Part print with two shaded views. Sizes in mm from the minimum x, y, z corner. A direction names the side the tool comes from. Give positions to 0.01 mm unless a question says otherwise; leave off trailing zeros. Write each loop counter-clockwise with the first axis right and the second up, starting at its lowest first coordinate (ties: lowest second). Pieces come first, ordered by that corner, then holes. Notation, with made-up numbers: (80, -26.75) - (119, -26.75) arc R19 ccw to (119, -4.75) - close; hole circle Ø6 at (26.25, 41.25). An arc over 180 degrees is marked (long way). Answer as a JSON object with one key per item and string values. Group by question number.
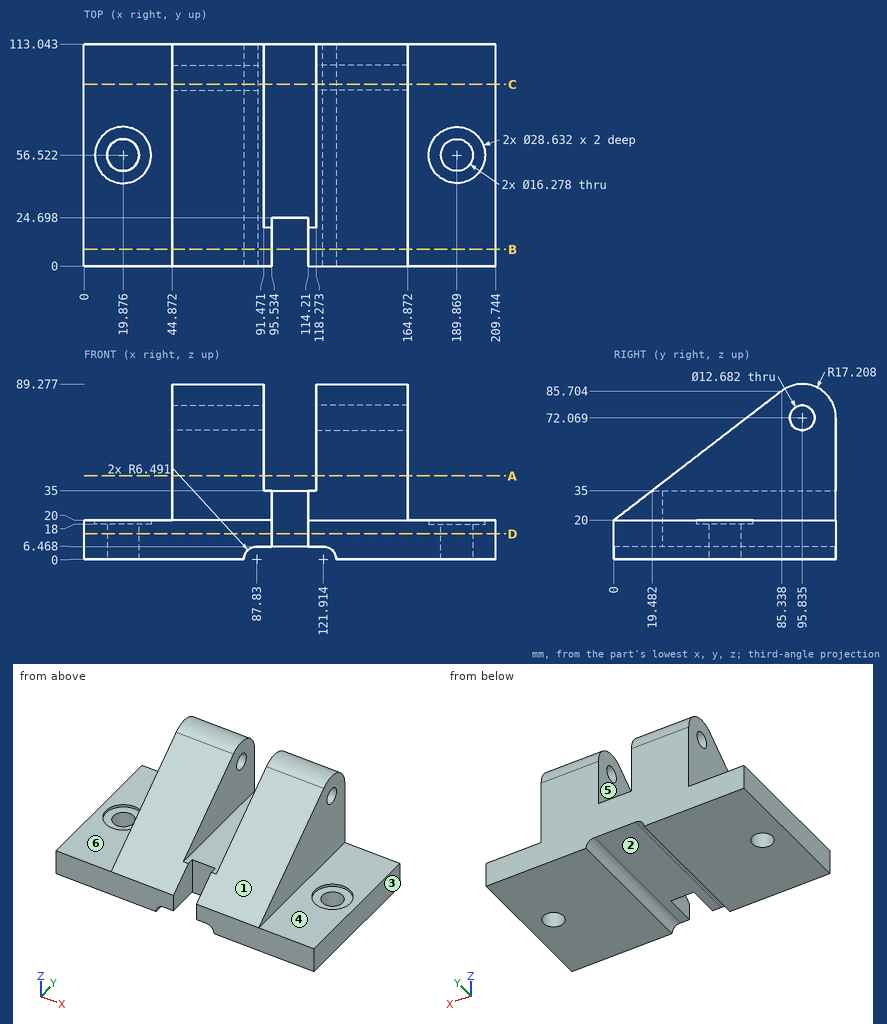
1) Drill centre lines: line 1 along X through (y, z) = (46, 38.5); line 2 along X through (y, z) = (57.5, 15) (1 decimal); line 3 along Z through (x, y) = (12.5, 103.5). Where is each one in solid material? Low to high. Write a range as from..to.
2) Drop flat-ended pins along their axis: P1, Ø1, axis at y = 87, z = 22.5, coming from the -X side; P2, Ø23, axis at x = 191.5, y = 63, coming from the +Z side; P3, Ø3, axis at y = 90.5, z = 67, coming from the +X side; P4, Ø10, axis at y = 101.5, z = 15.5, coming from the -X side. Give the stop position or say it passes through.
3) Saw through at D-D (z = 13). List the corners of the cut face in (x, y) (1 decimal).
4) Saw through at B-B (y = 8.5). List the corners of the cut face in (x, z) (1 decimal).
5) Saw through at C-C (y = 92.5). State how many separate pieces and enclosed holes the cut face has, and give its area (3 significant figures).
6) Two-plate mould, pull along X, no slides. Class the marked faces 1, 2 and 3: +X half, -X half, draft (parallel to the pull), parting line (faces both ways), or undercut.
7) Which spindle directions (+Z, -Z, +X, -X, +Y, -Y) get a long thin tool onto all of the face, cutting with end or side? Do the marked faces 4, 5 and 6. Say none if no direction does.
8) Saw through at A-A (z = 42.5). List the corners of the cut face in (x, y).
Checks:
{
 "1": {"line 1": "44.87..91.47, 118.27..164.87", "line 2": "0..11.8, 28..181.8, 197.9..209.7", "line 3": "0..20"},
 "2": {"P1": "x = 44.87", "P2": "z = 20", "P3": "x = 164.87", "P4": "x = 0"},
 "3": {"outline": "(0, 0) - (95.5, 0) - (95.5, 24.7) - (114.2, 24.7) - (114.2, 0) - (209.7, 0) - (209.7, 113) - (0, 113) - close; hole circle Ø16.3 at (19.9, 56.5); hole circle Ø16.3 at (189.9, 56.5)"},
 "4": {"outline": "(0, 0) - (81.3, 0) arc R6.5 cw to (88.4, 6.5) - (95.5, 6.5) - (95.5, 26.5) - (44.9, 26.5) - (44.9, 20) - (0, 20) - close; (114.2, 6.5) - (121.4, 6.5) arc R6.5 cw to (128.4, 0) - (209.7, 0) - (209.7, 20) - (164.9, 20) - (164.9, 26.5) - (114.2, 26.5) - close"},
 "5": {"separate pieces": "3", "enclosed holes": "0", "area": "9,730 mm2"},
 "6": {"face 1": "draft", "face 2": "undercut", "face 3": "+X half"},
 "7": {"face 4": "+Z, +X, +Y, -Y", "face 5": "+Z, +Y, -Y", "face 6": "+Z, -X, +Y, -Y"},
 "8": {"outline": "(44.87, 29.22) - (91.47, 29.22) - (91.47, 113.04) - (44.87, 113.04) - close; (118.27, 29.22) - (164.87, 29.22) - (164.87, 113.04) - (118.27, 113.04) - close"}
}
